Model file for the job. Use its own axes, mm. Face numbers are marked on the shaded views. A direction names the side the tool comes from. Coordinates: 2 decimals unless noted, no trailing zeros. Write each loop counter-clockwise with the first axis right and the second up, starting at its lowest first coordinate (ties: lowest second). Pieces come first, ordered by that corner, then holes. Notation, with made-up numbers: (50.25, 55.25) - (81.25, 55.25) arc R14 ccw to (81.25, 77.25) - close; hole circle Ø11 at (14, 40.5). An arc over 180 degrees is marked (long way). Put each result on its own line as item: value. Start each with the question number.
1. Which spindle directions (+Z, -Z, +X, -X, +Y, -Y) get a long thin tool onto all of the face, cutting with end or side? Do the marked faces 1, 2 and 3. Say none if no direction does.
2. Saw through at A-A, the plane y = 24. Write the cut outline in (x, z), plus the area to 3 significant figures.
3. Drill centre lines: L1, parallel to X at y = 20.5, z = 0.5; L2, parallel to Z at x = -5.5, y = 46; L3, parallel to Y at x = 3.5, z = 5.5. Where is each one in solid material? Low to high. Write a range as from..to.
4. Drop flat-ended pins along their axis: P1, Ø5, axis at x = -4.5, z = -3.5, coming from the -Y side; P2, Ø1.5, axis at x = 1, z = -1, coming from the -Y side; P3, Ø6, axis at x = 2.5, y = 44.5, coming from the +Z side; P4, Ø3, axis at x = 6, y = 26.5, coming from the -Z side. Give the stop position or say it passes through.
5. Saw through at B-B, the plane y = 30. Write the cut outline in (x, z), plus the area to 3 significant figures.
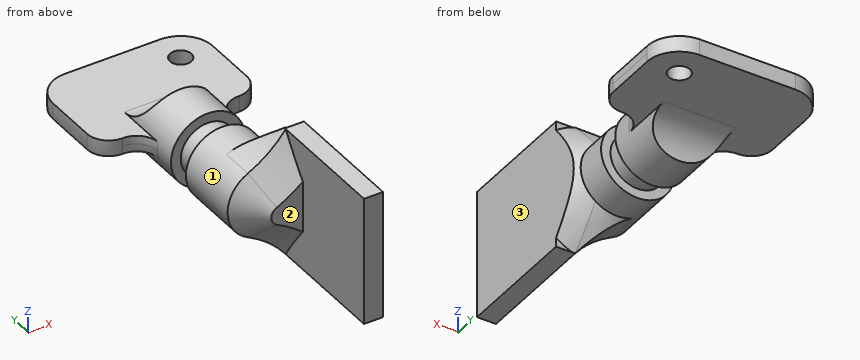
```python
from build123d import *

# Parameters (mm, degrees)
BOSS_EXTRUDE1_DEPTH      = 10
FILLET2_R                = 2
FILLET3_R                = 3
CUT_EXTRUDE1_DEPTH       = 49.473897211
CUT_EXTRUDE1_DEPTH_BACK  = 49.473897211
SKETCH3_R                = 1
BOSS_EXTRUDE2_DEPTH      = 6
BOSS_EXTRUDE2_DEPTH_BACK = 6
SKETCH4_W                = 1.78
SKETCH4_H                = 11.625349657
CHAMFER1_SIZE            = 3
FILLET4_START            = 23
FILLET4_DEPTH            = 2.747219164
FILLET4_START_2          = 25.747219164
FILLET4_2_DEPTH          = 2.878130593
CHAMFER2_SIZE            = 2.5


with BuildPart() as part:
    # Sketch1 → Revolve1 (revolve)
    with BuildSketch(Plane.XY):
        Polygon((-3.448914015, 37.765821371), (-3.448914015, 33.765821371), (-2.534753992, 33.765821371), (-2.534753992, 31.624967984), (-3.41766068, 31.624967984), (-3.41766068, 23), (0, 23), (0, 37.765821371), align=None)
    revolve(axis=Axis((0, 37.765821371, 0), (0, -1, 0)))

    # Sketch2 → Boss-Extrude1 (add)
    with BuildSketch(Plane(origin=(0, 37.765821371, 0), x_dir=(1, 0, 0), z_dir=(0, 1, 0))):
        with BuildLine():
            Line((3.366379046, 0.75), (-3.366379046, 0.75))
            ThreePointArc((-3.366379046, 0.75), (-3.448914015, 0), (-3.366379046, -0.75))
            Line((-3.366379046, -0.75), (3.366379046, -0.75))
            ThreePointArc((3.366379046, -0.75), (3.428218178, -0.37726384), (3.448914015, 0))
            ThreePointArc((3.448914015, 0), (3.428218178, 0.37726384), (3.366379046, 0.75))
        make_face()
        with BuildLine():
            Line((-3.366379046, 0.75), (-7.462405778, 0.75))
            ThreePointArc((-7.462405778, 0.75), (-7.5, 0), (-7.462405778, -0.75))
            Line((-7.462405778, -0.75), (-3.366379046, -0.75))
            ThreePointArc((-3.366379046, -0.75), (-3.448914015, 0), (-3.366379046, 0.75))
        make_face()
        with BuildLine():
            ThreePointArc((7.5, 0), (7.490595548, 0.375470813), (7.462405778, 0.75))
            Line((7.462405778, 0.75), (3.366379046, 0.75))
            ThreePointArc((3.366379046, 0.75), (3.428218178, 0.37726384), (3.448914015, 0))
            ThreePointArc((3.448914015, 0), (3.428218178, -0.37726384), (3.366379046, -0.75))
            Line((3.366379046, -0.75), (7.462405778, -0.75))
            ThreePointArc((7.462405778, -0.75), (7.490595548, -0.375470813), (7.5, 0))
        make_face()
    extrude(amount=BOSS_EXTRUDE1_DEPTH)

    # Fillet2
    # the kernel refuses this fillet: 2 mm, written as the material it adds along each edge
    with BuildSketch(Plane(origin=(0, 37.765821371, 0), x_dir=(-0.09803421101524086, 0, -0.9951830452085783), z_dir=(-0.9951830452085783, 0, 0.09803421101524086))) as fillet2_piece_1_section:
        with BuildLine():
            CenterArc((3.448914015 + FILLET2_R, FILLET2_R), FILLET2_R, 180, 90)
            Line((3.448914015 + FILLET2_R, 0), (3.448914015, 0))
            Line((3.448914015, 0), (3.448914015, FILLET2_R))
        make_face()
    fillet2_piece_1 = revolve(axis=Axis((0, 37.765821371, 0), (0, -1, 0)), revolution_arc=191.251965623, mode=Mode.PRIVATE)
    fillet2_piece_1 = split(fillet2_piece_1, bisect_by=Plane(origin=(0, 37.765821371, -0.75), z_dir=(0, 0, 1)), keep=Keep.TOP, mode=Mode.PRIVATE)
    fillet2_piece_1 = split(fillet2_piece_1, bisect_by=Plane(origin=(0, 37.765821371, 0.75), z_dir=(0, 0, -1)), keep=Keep.TOP, mode=Mode.PRIVATE)
    add(fillet2_piece_1)
    with BuildSketch(Plane(origin=(0, 37.765821371, 0), x_dir=(0.09800035789508027, 0, 0.9951863794548418), z_dir=(0.9951863794548418, 0, -0.09800035789508027))) as fillet2_piece_2_section:
        with BuildLine():
            CenterArc((3.448914015 + FILLET2_R, FILLET2_R), FILLET2_R, 180, 90)
            Line((3.448914015 + FILLET2_R, 0), (3.448914015, 0))
            Line((3.448914015, 0), (3.448914015, FILLET2_R))
        make_face()
    fillet2_piece_2 = revolve(axis=Axis((0, 37.765821371, 0), (0, -1, 0)), revolution_arc=95.624033786, mode=Mode.PRIVATE)
    fillet2_piece_2 = split(fillet2_piece_2, bisect_by=Plane(origin=(0, 37.765821371, 0.75), z_dir=(0, 0, -1)), keep=Keep.TOP, mode=Mode.PRIVATE)
    add(fillet2_piece_2)
    with BuildSketch(Plane(origin=(0, 37.765821371, 0), x_dir=(-1, 0, 0), z_dir=(0, 0, 1))) as fillet2_piece_3_section:
        with BuildLine():
            CenterArc((3.448914015 + FILLET2_R, FILLET2_R), FILLET2_R, 180, 90)
            Line((3.448914015 + FILLET2_R, 0), (3.448914015, 0))
            Line((3.448914015, 0), (3.448914015, FILLET2_R))
        make_face()
    fillet2_piece_3 = revolve(axis=Axis((0, 37.765821371, 0), (0, -1, 0)), revolution_arc=95.624033786, mode=Mode.PRIVATE)
    fillet2_piece_3 = split(fillet2_piece_3, bisect_by=Plane(origin=(0, 37.765821371, -0.75), z_dir=(0, 0, 1)), keep=Keep.TOP, mode=Mode.PRIVATE)
    add(fillet2_piece_3)
    # the kernel refuses this fillet: 2 mm, written as the material it takes off along each edge
    with BuildSketch(Plane(origin=(0, 37.765821371, 0), x_dir=(-0.7201079494948177, 0, -0.6938620475817721), z_dir=(0.6938620475817721, 0, -0.7201079494948177))) as fillet2_2_piece_1:
        with BuildLine():
            CenterArc((7.5 - FILLET2_R, FILLET2_R), FILLET2_R, 270, 90)
            Line((7.5, FILLET2_R), (7.5, 0))
            Line((7.5, 0), (7.5 - FILLET2_R, 0))
        make_face()
    revolve(axis=Axis((0, 37.765821371, 0), (0, 1, 0)), revolution_arc=87.873212667, mode=Mode.SUBTRACT)
    with BuildSketch(Plane(origin=(0, 37.765821371, 0), x_dir=(0.7201079494948216, 0, 0.6938620475817678), z_dir=(-0.6938620475817678, 0, 0.7201079494948216))) as fillet2_2_piece_2:
        with BuildLine():
            CenterArc((7.5 - FILLET2_R, FILLET2_R), FILLET2_R, 270, 90)
            Line((7.5 - FILLET2_R, 0), (7.5, 0))
            Line((7.5, 0), (7.5, FILLET2_R))
        make_face()
    revolve(axis=Axis((0, 37.765821371, 0), (0, 1, 0)), revolution_arc=87.873212667, mode=Mode.SUBTRACT)

    # Fillet3
    # the kernel refuses this fillet: 3 mm, written as the material it adds along each edge
    with BuildSketch(Plane(origin=(10.866379046, 37.765821371, -0.75), x_dir=(0, 1, 0), z_dir=(-1, 0, 0))) as fillet3_piece_1_section:
        with BuildLine():
            CenterArc((FILLET3_R, FILLET3_R), FILLET3_R, 180, 90)
            Line((0, FILLET3_R), (0, 0))
            Line((0, 0), (FILLET3_R, 0))
        make_face()
    fillet3_piece_1 = extrude(amount=21.732758092, mode=Mode.PRIVATE)
    fillet3_piece_1 = fillet3_piece_1 & Plane(origin=(0, 37.765821371, 0), x_dir=(-1, 0, 0), z_dir=(0, -1, 0)) * Cylinder(3.448914015, 56, mode=Mode.PRIVATE)
    add(fillet3_piece_1)
    with BuildSketch(Plane(origin=(10.866379046, 37.765821371, 0.75), x_dir=(0, 1, 0), z_dir=(-1, 0, 0))) as fillet3_piece_2_section:
        with BuildLine():
            CenterArc((FILLET3_R, -FILLET3_R), FILLET3_R, 90, 90)
            Line((0, -FILLET3_R), (0, 0))
            Line((0, 0), (FILLET3_R, 0))
        make_face()
    fillet3_piece_2 = extrude(amount=21.732758092, mode=Mode.PRIVATE)
    fillet3_piece_2 = fillet3_piece_2 & Plane(origin=(0, 37.765821371, 0), x_dir=(-1, 0, 0), z_dir=(0, -1, 0)) * Cylinder(3.448914015, 56, mode=Mode.PRIVATE)
    add(fillet3_piece_2)
    # the kernel refuses this fillet: 3 mm, written as the material it takes off along each edge
    with BuildSketch(Plane(origin=(0, 47.765821371, 0), x_dir=(-0.4534410859899706, 0, -0.8912862511764871), z_dir=(0.8912862511764871, 0, -0.4534410859899706))) as fillet3_2_piece_1:
        with BuildLine():
            CenterArc((7.5 - FILLET3_R, -FILLET3_R), FILLET3_R, 0, 90)
            Line((7.5 - FILLET3_R, 0), (7.5, 0))
            Line((7.5, 0), (7.5, -FILLET3_R))
        make_face()
    revolve(axis=Axis((0, 47.765821371, 0), (0, 1, 0)), revolution_arc=126.070648523, mode=Mode.SUBTRACT)
    with BuildSketch(Plane(origin=(0, 47.765821371, 0), x_dir=(0.4534410859901425, 0, -0.8912862511763997), z_dir=(-0.8912862511763997, 0, -0.4534410859901425))) as fillet3_2_piece_2:
        with BuildLine():
            CenterArc((7.5 - FILLET3_R, FILLET3_R), FILLET3_R, 270, 90)
            Line((7.5, FILLET3_R), (7.5, 0))
            Line((7.5, 0), (7.5 - FILLET3_R, 0))
        make_face()
    revolve(axis=Axis((0, 47.765821371, 0), (0, -1, 0)), revolution_arc=126.070648523, mode=Mode.SUBTRACT)

    # Sketch3 → Cut-Extrude1 (cut, two sides: drawn at the far end of the back side and taken through both)
    with BuildSketch(Plane.XY.offset(-CUT_EXTRUDE1_DEPTH_BACK)):
        with Locations((4.462405778, 44.765821371)):
            Circle(SKETCH3_R)
    extrude(amount=CUT_EXTRUDE1_DEPTH + CUT_EXTRUDE1_DEPTH_BACK, mode=Mode.SUBTRACT)

    # Sketch4 → Boss-Extrude2 (add, two sides: drawn at the far end of the back side and taken through both)
    with BuildSketch(Plane.XY.offset(-BOSS_EXTRUDE2_DEPTH_BACK)):
        with Locations((2.92, 19.812674829)):
            Rectangle(SKETCH4_W, SKETCH4_H)
    extrude(amount=BOSS_EXTRUDE2_DEPTH + BOSS_EXTRUDE2_DEPTH_BACK)

    # Chamfer1
    # the kernel refuses this chamfer: 3 mm, written as the material it adds along each edge
    with BuildSketch(Plane(origin=(0, 25.625349657, 0), x_dir=(-0.9999950652018582, 0, -0.003141587485879368), z_dir=(-0.003141587485879368, 0, 0.9999950652018582))) as chamfer1_piece_1_section:
        Polygon((3.41766068, -CHAMFER1_SIZE), (3.41766068 + CHAMFER1_SIZE, 0), (3.41766068, 0), align=None)
    chamfer1_piece_1 = revolve(axis=Axis((0, 25.625349657, 0), (0, -1, 0)), revolution_arc=359.64, mode=Mode.PRIVATE)
    chamfer1_piece_1 = split(chamfer1_piece_1, bisect_by=Plane(origin=(2.03, 25.625349657, 0), z_dir=(1, 0, 0)), keep=Keep.TOP, mode=Mode.PRIVATE)
    chamfer1_piece_1 = split(chamfer1_piece_1, bisect_by=Plane(origin=(0, 25.625349657, -6), z_dir=(0, 0, 1)), keep=Keep.TOP, mode=Mode.PRIVATE)
    chamfer1_piece_1 = split(chamfer1_piece_1, bisect_by=Plane(origin=(3.81, 25.625349657, 0), z_dir=(-1, 0, 0)), keep=Keep.TOP, mode=Mode.PRIVATE)
    chamfer1_piece_1 = split(chamfer1_piece_1, bisect_by=Plane(origin=(0, 25.625349657, 6), z_dir=(0, 0, -1)), keep=Keep.TOP, mode=Mode.PRIVATE)
    add(chamfer1_piece_1)

    # Fillet4: read off the stored shape, not the designer's step
    # Fillet4 outline → Fillet4 (add)
    with BuildSketch(Plane(origin=(0, 0, 0), x_dir=(1, 0, 0), z_dir=(0, 1, 0)).offset(FILLET4_START)):
        with BuildLine():
            Line((2.03, 2.749455314), (2.03, 6))
            ThreePointArc((2.03, 6), (0.428490728, 4.324777263), (-1.515640098, 3.063207407))
            ThreePointArc((-1.515640098, 3.063207407), (0.301250097, 3.404357928), (2.03, 2.749455314))
        make_face()
        with BuildLine():
            ThreePointArc((2.03, -2.749455314), (0.301250097, -3.404357928), (-1.515640098, -3.063207407))
            ThreePointArc((-1.515640098, -3.063207407), (0.428490728, -4.324777263), (2.03, -6))
            Line((2.03, -6), (2.03, -2.749455314))
        make_face()
    extrude(amount=FILLET4_DEPTH)

    # Fillet4 2 outline → Fillet4 2 (add)
    with BuildSketch(Plane(origin=(0, 0, 0), x_dir=(1, 0, 0), z_dir=(0, 1, 0)).offset(FILLET4_START_2)):
        with BuildLine():
            Line((2.03, 2.749455314), (2.03, 6))
            ThreePointArc((2.03, 6), (0.428490728, 4.324777263), (-1.515640098, 3.063207407))
            ThreePointArc((-1.515640098, 3.063207407), (0.301250097, 3.404357928), (2.03, 2.749455314))
        make_face()
        with BuildLine():
            ThreePointArc((2.03, -2.749455314), (0.301250097, -3.404357928), (-1.515640098, -3.063207407))
            ThreePointArc((-1.515640098, -3.063207407), (0.428490728, -4.324777263), (2.03, -6))
            Line((2.03, -6), (2.03, -2.749455314))
        make_face()
    extrude(amount=FILLET4_2_DEPTH)

    # Fillet4 3 outline → Fillet4 3 (revolve, cut)
    with BuildSketch(Plane.XY):
        Polygon((6.334106093, 28.625349757), (3.41766068, 28.625349757), (6.41766068, 25.625349657), (6.41766068, 28.62535645), align=None)
    revolve(axis=Axis((0, 0, 0), (0, 1, 0)), mode=Mode.SUBTRACT)

    # Chamfer2
    chamfer2_edges = [part.edges().sort_by_distance(p)[0] for p in [
        (-2.903476201, 23, 1.80283956),
        (0.428490728, 23, -4.324777263),
        (0.428490728, 23, 4.324777263),
    ]]
    chamfer(chamfer2_edges, length=CHAMFER2_SIZE)


solid = part.part
```
Final values:
1. face 1: none
1. face 2: +Z, -Z, -X, -Y
1. face 3: +Z, -Z, +X, -Y
2. outline: (-0.85, -1.72) arc R11.5 cw to (2.03, -3.75) - (2.03, -6) - (3.81, -6) - (3.81, 6) - (2.03, 6) - (2.03, 3.75) arc R11.5 cw to (-0.85, 1.72) arc R1.92 ccw to start
2. area: 39.1 mm²
3. L1: x = 2.03..3.81
3. L2: z = -0.75..0.75
3. L3: y = 14..25.63
4. P1: stops at y = 25.28
4. P2: stops at y = 23
4. P3: stops at z = 0.75
4. P4: passes through
5. outline: circle Ø6.84 at (0, 0)
5. area: 36.7 mm²
